Work out the finished part from the listing and answer in its coordinate system (mm). Give positions to 0.01 mm unless a question says otherwise; leave off trailing zeros. Put each result on its own line as item: value.
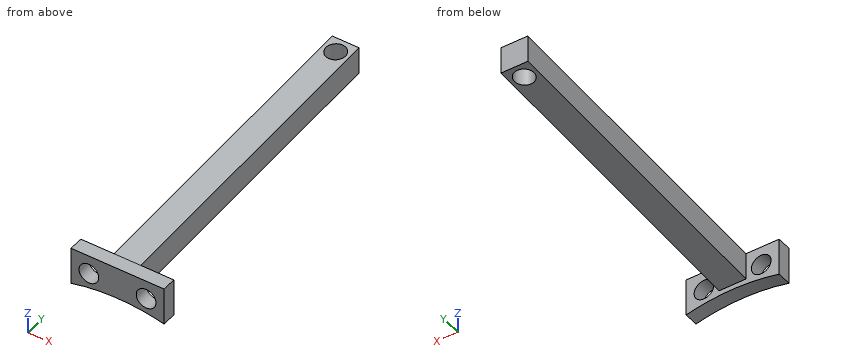
```python
from build123d import *

# Parameters (mm, degrees)
BOSS_EXTRUDE1_DEPTH     = 2
SKETCH2_R               = 1.375
CUT_EXTRUDE1_DEPTH      = 2
CUT_EXTRUDE3_DEPTH      = 47.745974282
CUT_EXTRUDE3_DEPTH_BACK = 47.745974282
SKETCH12_R              = 1.375


with BuildPart() as part:
    # Sketch1 → Boss-Extrude1 (new body)
    with BuildSketch(Plane(origin=(0, 0, 0), x_dir=(1, 0, 0), z_dir=(0, 1, 0))):
        with BuildLine():
            Line((-6.5, 0), (6.5, 0))
            Line((6.5, 0), (6.5, 5.19))
            add(Edge.make_bspline(
                [(-6.5, 5.19), (0, 3.63), (6.5, 5.19)],
                knots=[0, 0, 0, 1, 1, 1], degree=2))
            Line((-6.5, 5.19), (-6.5, 0))
        make_face()
    extrude(amount=BOSS_EXTRUDE1_DEPTH)

    # Sketch2 → Cut-Extrude1 (cut)
    with BuildSketch(Plane(origin=(0, 2, 0), x_dir=(1, 0, 0), z_dir=(0, 1, 0))):
        with Locations(Location((-4, 2.595, 0), (0, 0, 270))):
            Circle(SKETCH2_R)
        with Locations(Location((4, 2.595, 0), (0, 0, 270))):
            Circle(SKETCH2_R)
    extrude(amount=-CUT_EXTRUDE1_DEPTH, mode=Mode.SUBTRACT)

    # Sketch4 → Loft2 section 0
    with BuildSketch(Plane(origin=(0, 2, 0), x_dir=(1, 0, 0), z_dir=(0, 1, 0))):
        with BuildLine():
            Line((-1.875, 3.75), (1.875, 3.75))
            Line((1.875, 3.75), (1.875, 0))
            Line((1.875, 0), (-1.875, 0))
            Line((-1.875, 0), (-1.875, 3.75))
        make_face()
    # Sketch6 → Loft2 section 1
    with BuildSketch(Plane(origin=(0, 46, 0), x_dir=(1, 0, 0), z_dir=(0, 1, 0))):
        with BuildLine():
            Line((-1.875, 1), (1.875, 1))
            Line((1.875, 1), (1.875, -2.75))
            Line((1.875, -2.75), (-1.875, -2.75))
            Line((-1.875, -2.75), (-1.875, 1))
        make_face()
    loft()

    # Sketch12 → Cut-Extrude3 (cut, two sides: drawn at the far end of the back side and taken through both)
    with BuildSketch(Plane.XY.offset(-CUT_EXTRUDE3_DEPTH_BACK)):
        with Locations(Location((0, 44, 0), (0, 0, 90))):
            Circle(SKETCH12_R)
    extrude(amount=CUT_EXTRUDE3_DEPTH + CUT_EXTRUDE3_DEPTH_BACK, mode=Mode.SUBTRACT)


solid = part.part
```
(1) Section A-A, the plane z = -2.5 is taken. Count the separate pieces of the cut face and the enclosed holes in it, then the cut area to 3 significant figures.
Geometry check:
separate pieces: 3
enclosed holes: 0
area: 90.0 mm²
(2) Given pin 1 (1.5 mm diameter, centred on x = -0.5, y = 28.5, fed in from +Z); pin 2 (1 mm diameter, centred on x = 2.5, y = 0.5, fed in from +Z); pin 3 (2 mm diameter, centred on y = 23.5, z = -3, fed in from +X) (3 decimals), each flat-ended and moving along its own axis, determine where each tip first touches the part or whether it passes through.
Geometry check:
pin 1: stops at z = 1.7
pin 2: stops at z = 0
pin 3: stops at x = 1.875
(3) Straight lines are drawn through the part: line 1 (X direction, y = 44, z = 1.45) (3 decimals); line 2 (X direction, y = 16, z = 0) (3 decimals); line 3 (Y direction, x = 5, z = -3.75). For each, find the intervals that lie inside material, in ascending order.
Geometry check:
line 1: x = -1.875 to -1.375, 1.375 to 1.875
line 2: x = -1.875 to 1.875
line 3: y = 0 to 2
